Solid Edge part; units mm, degrees
sketch "Sketch1" plane through (0, 0, 0) normal (0, -1, 0) x (1, 0, 0)
  arc A0 (30, 30) -> (90, 30) centre (60, 30) cw
  line L0 (120, 30) -> (90, 30)
  line L1 (120, 0) -> (120, 30)
  line L2 (0, 0) -> (120, 0)
  line L3 (0, 0) -> (0, 30)
  line L4 (0, 30) -> (30, 30)
extrude "Protrusion1" add sketch "Sketch1" against normal blind 45
sketch "Sketch2" plane through (60, 0, 30) normal (0, -1, 0) x (1, 0, 0)
  circle A0 centre (0, 0) radius 10
extrude "ExtrudedCutout_1" cut sketch "Sketch2" against normal blind 214.5997
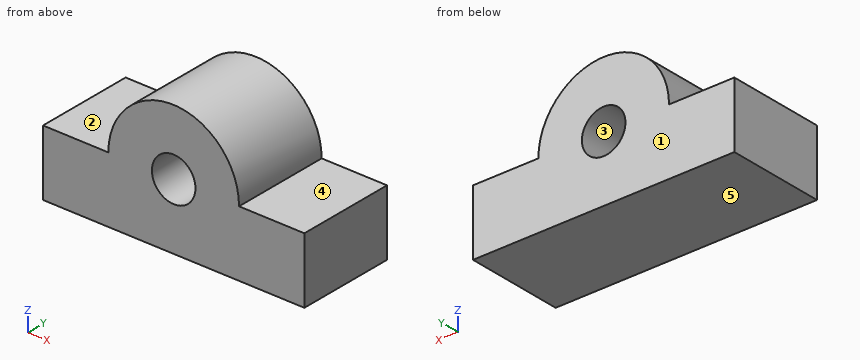
Source: CAD feature listing. Evaluate the final solid. Frame: model axes, mm. Face numbers are marked on the shaded views. A direction names the side the tool comes from. Round coordinates to 2 decimals unless told otherwise and drop trailing zeros. Loops run counter-clockwise (first coordinate to the right, second up) from the corner with the lowest first, then second, coordinate; pieces in that order, holes last. Notation, with made-up numbers: (81, 85.5) - (130, 85.5) arc R16 cw to (130, 91.5) - close; hole circle Ø2 at (61.25, 18.5). An arc over 180 degrees is marked (long way). Write item = value, one per line. Start each with the question number.
(1) Section query B-B, the plane x = 60. Output: boundary loops of the cut face in (y, z).
(2) Section query C-C, the plane z = 22. Output: boundary loops of the cut face in (x, y).
(3) Section query A-A, the plane y = 30. Output: boundary loops of the cut face in (x, z), plus the area to 3 significant figures.
(4) Ray query, line 1 along Z through (x, y) = (60, 14); line 2 along Z through (x, y) = (6, 13); line 3 along Z through (x, y) = (65.5, 28). Return the intervals inside material, ascending. Write a range as from..to.
(5) Pin query (flat end, axial travel): pin 1 (9 mm diameter, centred on x = 9.5, y = 13, fed in from +Z); pin 2 (2 mm diameter, centred on y = 11.5, z = 42.5, fed in from -X); pin 3 (1.5 mm diameter, centred on y = 19.5, z = 41.5, fed in from +X); pin 4 (8 mm diameter, centred on x = 101.5, y = 40.5, fed in from -Z). Return the tip coordinate at first contact, or that it passes through.
(6) Set-up query: the marked faces 1 and 2. Return all of +Z, -Z, +X, -X, +Y, -Y with unobstructed straight access to the full face (end or side cutting, diameter ignored); none if empty.
(7) Section query D-D, the plane z = 42. Output: boundary loops of the cut face in (x, y).
(8) Pull-direction query (Z, two-part tool) for the marked faces 3, 4 and 5; classes: +Z half, -Z half, draft (parallel to the pull), parting line (faces both ways), or undercut.
Conclusion:
q1.outline = (0, 0) - (45, 0) - (45, 20) - (0, 20) - close; (0, 40) - (45, 40) - (45, 60) - (0, 60) - close
q2.outline = (0, 0) - (54, 0) - (54, 45) - (0, 45) - close; (66, 0) - (120, 0) - (120, 45) - (66, 45) - close
q3.outline = (0, 0) - (120, 0) - (120, 30) - (90, 30) arc R30 ccw to (30, 30) - (0, 30) - close; hole circle Ø20 at (60, 30)
q3.area = 4,700 mm2
q4.line_1 = 0..20, 40..60
q4.line_2 = 0..30
q4.line_3 = 0..21.65, 38.35..59.49
q5.pin_1 = 30
q5.pin_2 = 32.29
q5.pin_3 = 88.01
q5.pin_4 = 0
q6.face_1 = +Z, -Z, +X, -X, +Y
q6.face_2 = +Z, -X, +Y, -Y
q7.outline = (32.5, 0) - (87.5, 0) - (87.5, 45) - (32.5, 45) - close
q8.face_3 = undercut
q8.face_4 = +Z half
q8.face_5 = -Z half
